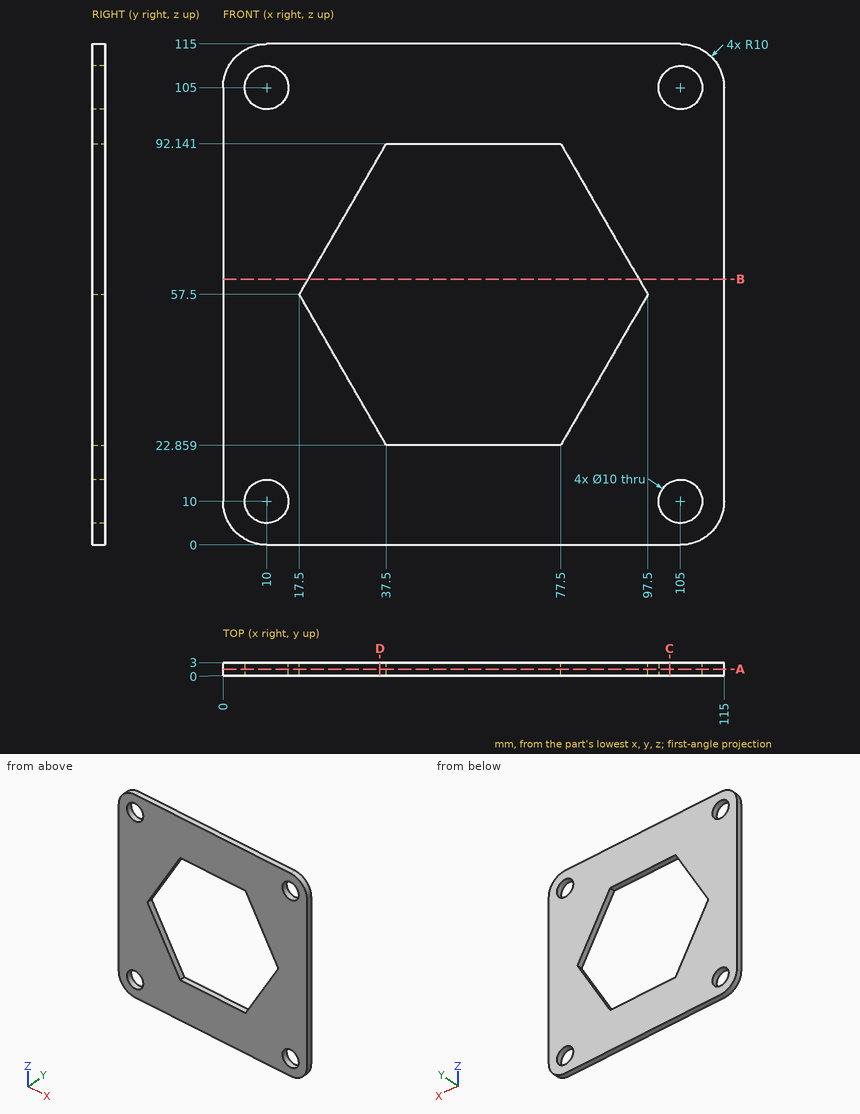
Verification items for this drawing (mm, ordinates from the low corner). Give positions to 0.01 mm unless a question says otherwise; leave off trailing zeros. Write each loop counter-clockwise with the first axis right and the second up, starting at its lowest first coordinate (ties: lowest second). Pieces come first, ordered by that corner, then holes. Notation, with made-up numbers: (53.25, 76) -> (82.25, 76) arc R16 cw to (82.25, 82) -> close; hole circle Ø5 at (20, 28). An arc over 180 degrees is marked (long way). Use one line per item in the form item = value.
Item 1: Sectioned sample at C-C on x = 102.5. Enter the section's corners in (y, z).
Results list:
outline = (0, 0) -> (3, 0) -> (3, 5.67) -> (0, 5.67) -> close; (0, 14.33) -> (3, 14.33) -> (3, 100.67) -> (0, 100.67) -> close; (0, 109.33) -> (3, 109.33) -> (3, 115) -> (0, 115) -> close
Item 2: Sectioned sample at D-D on x = 36. Enter the section's corners in (y, z), plus the area to 3 significant figures.
Results list:
outline = (0, 0) -> (3, 0) -> (3, 25.46) -> (0, 25.46) -> close; (0, 89.54) -> (3, 89.54) -> (3, 115) -> (0, 115) -> close
area = 153 mm2
Item 3: Sectioned sample at B-B on z = 61. Enter the section's corners in (x, y), plus the area to 3 significant figures.
Results list:
outline = (0, 0) -> (19.52, 0) -> (19.52, 3) -> (0, 3) -> close; (95.48, 0) -> (115, 0) -> (115, 3) -> (95.48, 3) -> close
area = 117 mm2
Item 4: Sectioned sample at A-A on y = 1.55. Enter the section's corners in (x, z), plus the area to 3 significant figures.
Results list:
outline = (0, 10) arc R10 ccw to (10, 0) -> (105, 0) arc R10 ccw to (115, 10) -> (115, 105) arc R10 ccw to (105, 115) -> (10, 115) arc R10 ccw to (0, 105) -> close; hole circle Ø10 at (10, 10); hole circle Ø10 at (10, 105); hole (17.5, 57.5) -> (37.5, 22.86) -> (77.5, 22.86) -> (97.5, 57.5) -> (77.5, 92.14) -> (37.5, 92.14) -> close; hole circle Ø10 at (105, 10); hole circle Ø10 at (105, 105)
area = 8,670 mm2
Item 5: Depth check by flat-ended pin: pin 1 Ø11.5 at (x, z) = (10, 105) entering from +Y. Enter the tip coordinate at first touch or a pass-through.
Results list:
pin_1 = 3
Item 6: Scan lines: line 1 (X direction, y = 1.3, z = 10); line 2 (Z direction, x = 70.5, y = 2.75); line 3 (X direction, y = 2.15, z = 6). Record each from-to range of solid material in increasing order.
Results list:
line_1 = 0 to 5, 15 to 100, 110 to 115
line_2 = 0 to 22.86, 92.14 to 115
line_3 = 0.83 to 7, 13 to 102, 108 to 114.17
